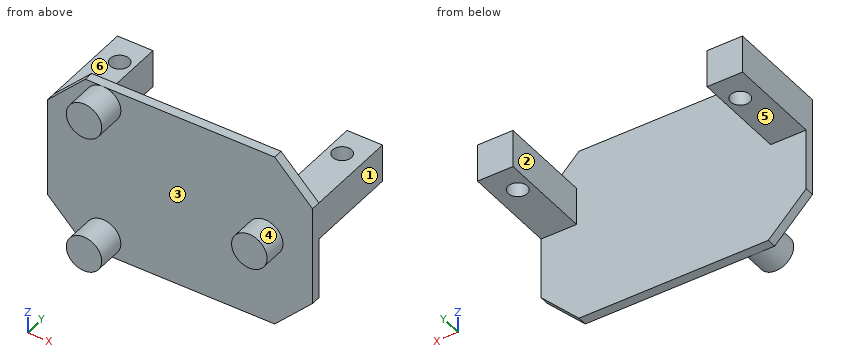
Autodesk Inventor part; units mm, degrees
ref_plane "YZ Plane" through (0, 0, 0) normal (1, 0, 0) x (0, 1, 0)
ref_plane "XZ Plane" through (0, 0, 0) normal (0, 1, 0) x (-1, 0, 0)
ref_plane "XY Plane" through (0, 0, 0) normal (0, 0, 1) x (1, 0, 0)
sketch "Sketch1" plane through (0, 0, 0) normal (0, 1, 0) x (-1, 0, 0)
  line L0 (56, 0) -> (0, 0) construction
  line L1 (0, 0) -> (0, -37) construction
  line L2 (0, -37) -> (56, -37) construction
  line L3 (56, -37) -> (56, 0) construction
  line L4 (56, 0) -> (48, 0) construction
  line L5 (48, 0) -> (48, -8) construction
  line L6 (48, -8) -> (56, -8) construction
  line L7 (56, -8) -> (56, 0) construction
  line L8 (56, -37) -> (48, -37) construction
  line L9 (48, -37) -> (48, -29) construction
  line L10 (48, -29) -> (56, -29) construction
  line L11 (56, -29) -> (56, -37) construction
  line L12 (0, 0) -> (8, 0) construction
  line L13 (8, 0) -> (8, -8) construction
  line L14 (8, -8) -> (0, -8) construction
  line L15 (0, -8) -> (0, 0) construction
  line L16 (0, -37) -> (8, -37) construction
  line L17 (8, -37) -> (8, -29) construction
  line L18 (8, -29) -> (0, -29) construction
  line L19 (0, -29) -> (0, -37) construction
  line L20 (48, 0) -> (56, -8)
  line L21 (56, -29) -> (48, -37)
  line L22 (8, -37) -> (0, -29)
  line L23 (8, 0) -> (0, -8)
  line L24 (56, -8) -> (56, -29)
  line L25 (48, -37) -> (8, -37)
  line L26 (0, -29) -> (0, -8)
  line L27 (8, 0) -> (48, 0)
  dimension "d0" = 56
  dimension "d1" = 37
  dimension "d2" = 8
  dimension "d3" = 8
  dimension "d4" = 8
  dimension "d5" = 8
  dimension "d6" = 8
  dimension "d7" = 8
  dimension "d8" = 8
  dimension "d9" = 8
extrude "Extrusion1" add sketch "Sketch1" along normal blind 2
sketch "Sketch2" plane through (0, 2, 0) normal (0, 1, 0) x (1, 0, 0)
  line L0 (-56, 29) -> (-56, 8)
  line L1 (-56, 8) -> (-48.5, 8)
  line L2 (-48.5, 8) -> (-48.5, 16)
  line L3 (-48.5, 16) -> (-56, 16)
  line L4 (-56, 16) -> (-56, 8)
  line L5 (-8, 0) -> (0, 8)
  line L6 (0, 8) -> (-7.5, 8)
  line L7 (-7.5, 8) -> (-7.5, 16)
  line L8 (-7.5, 16) -> (0, 16)
  line L9 (0, 16) -> (0, 8)
  point P0 (0, 0)
  dimension "d12" = 8
  dimension "d13" = 7.5
  dimension "d14" = 8
  dimension "d15" = 7.5
extrude "Extrusion2" add sketch "Sketch2" along normal blind 20
sketch "Sketch3" plane through (-56, 2, -8) normal (0, 0, 1) x (1, 0, 0)
  circle A0 centre (4.5, 14) radius 2
  line L0 (8, 0) -> (48, 0)
  line L1 (7.5, 0) -> (7.5, 20)
  circle A1 centre (51.5, 14) radius 2
  line L2 (48.5, 0) -> (48.5, 20)
  point P0 (56, -2)
  dimension "d18" = 14
  dimension "d19" = 3
  dimension "d20" = 4
  dimension "d21" = 14
  dimension "d22" = 3
  dimension "d23" = 4
extrude "Extrusion3" cut sketch "Sketch3" against normal through all
sketch "Sketch4" plane through (0, 0, 0) normal (0, -1, 0) x (1, 0, 0)
  circle A0 centre (-10, -18.5) radius 3.75
  line L0 (0, -8) -> (0, -29)
  line L1 (-48, 0) -> (-8, 0)
  circle A1 centre (-44.25, -3.75) radius 3.75
  circle A2 centre (-44.25, -33.25) radius 3.75
  line L2 (-56, -29) -> (-56, -8)
  point P0 (0, 0)
  dimension "d26" = 7.5
  dimension "d27" = 10
  dimension "d28" = 18.5
  dimension "d29" = 7.5
  dimension "d30" = 7.5
  dimension "d31" = 29.5
  dimension "d32" = 3.75
  dimension "d33" = 11.75
  dimension "d34" = 11.75
extrude "Extrusion4" add sketch "Sketch4" along normal blind 6 contours A1 | A2
extrude "Extrusion5" add sketch "Sketch4" along normal blind 5 contours A0
properties part number "RCT-P002_servo_plate_mount"
Can you work these out from the model? Positions are in its coordinate system, mm. Face numbers are marked on the shaded views. A direction names the side the tool comes from. Give positions to 0.01 mm unless a question says otherwise; leave off trailing zeros. Order: outer loops, then holes, each group sorted by start corner. A loop starts at its lowest first (then second) coordinate and runs counter-clockwise, first axis right, second up. Notation, with made-up numbers: M 4.25,79 L 19.25,79 A30 ccw 19.25,111 Z; hole C -15.75,59 d5. An arc over 180 degrees is marked long. Write item = value, one per line. Start each with the question number.
Q1. Will these pins go through, and if not, where does the flat tip stop? pin 1 Ø2 at (x, z) = (-16, -23) entering from -Y; pin 2 Ø8 at (x, z) = (-10.5, -18.5) entering from -Y; pin 3 Ø6 at (x, y) = (-51, 7) entering from +Z.
Q2. I need wall thicknesses on probe 1 along Y at (x, z) = (-4.5, -10); probe 2 along X at (y, z) = (18.5, -12); probe 3 along Y at (x, z) = (-29, -26). Which ranges of each line are inside material? Lowest first, please. Write a range as [from, to].
Q3. Suppose I cut it at A-A (y = 16). Write out the boundary of the cut face in (x, z).
Q4. Suppose I cut it at D-D (x = -10). Write out the boundary of the cut face in (y, z).
Q5. For the marked faces 4, 5 and 6, which set-ups out of +Z, -Z, +X, -X, +Y, -Y let a thin tool reach every point of the face, with its end or its side?
Q6. Suppose I cut it at B-B (x = -51.5). Write out the boundary of the cut face in (y, z), plus the area to 3 significant figures.
Q7. We'd pull the mould along X, two halves only. Please class the marked faces 1, 2 and 3: pulls with the +X half, pulls with the -X half, needs draft (parallel to the pull), parting line crosses it, or undercut.
Q8. Suppose I cut it at C-C (z = -33.25). Write out the boundary of the cut face in (x, y).
Check result:
q1.pin_1 = 0
q1.pin_2 = -5
q1.pin_3 = -8
q2.probe_1 = [0, 14], [18, 22]
q2.probe_2 = [-56, -48.5], [-7.5, 0]
q2.probe_3 = [0, 2]
q3.outline = M -56,-16 L -53.5,-16 L -53.5,-8 L -56,-8 Z; M -49.5,-16 L -48.5,-16 L -48.5,-8 L -49.5,-8 Z; M -7.5,-16 L -6.5,-16 L -6.5,-8 L -7.5,-8 Z; M -2.5,-16 L 0,-16 L 0,-8 L -2.5,-8 Z
q4.outline = M -5,-22.25 L 0,-22.25 L 0,-37 L 2,-37 L 2,0 L 0,0 L 0,-14.75 L -5,-14.75 Z
q5.face_4 = -Y
q5.face_5 = -Z, +X, -X, +Y
q5.face_6 = +Z, +X, -X, +Y
q6.outline = M 0,-33.5 L 2,-33.5 L 2,-16 L 14,-16 L 14,-8 L 2,-8 L 2,-3.5 L 0,-3.5 Z; M 18,-16 L 22,-16 L 22,-8 L 18,-8 Z
q6.area = 188 mm2
q7.face_1 = pulls with the +X half
q7.face_2 = undercut
q7.face_3 = needs draft
q8.outline = M -51.75,0 L -48,0 L -48,-6 L -40.5,-6 L -40.5,0 L -4.25,0 L -4.25,2 L -51.75,2 Z
